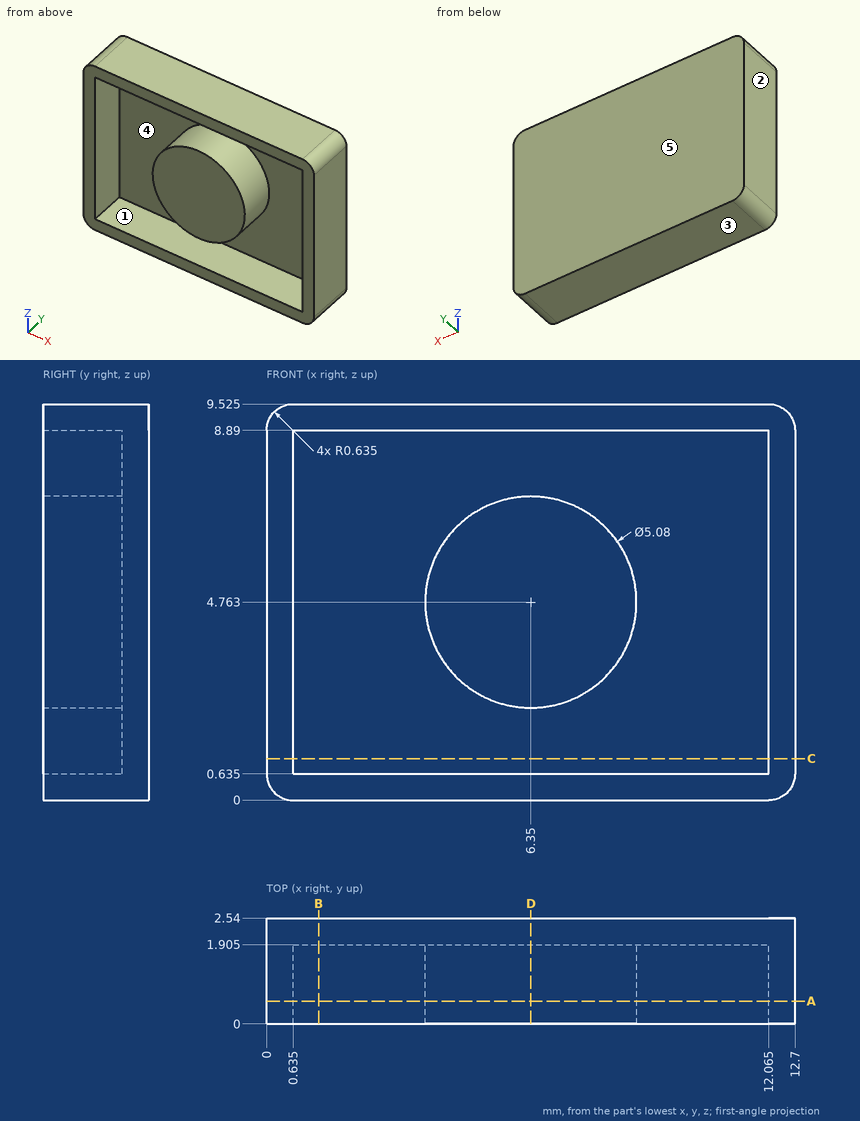
Print and shaded views of the part. All mm, measured from the part's lowest x, y and z. A direction names the side the tool comes from. Give positions to 0.01 mm unless a question says otherwise; leave off trailing zeros. Write each loop counter-clockwise with the first axis right and the second up, starting at its lowest first coordinate (ties: lowest second). Pieces come first, ordered by that corner, then holes. Notation, with made-up numbers: (-33.5, 82) -> (-12.5, 82) arc R16 cw to (-12.5, 108) -> close; hole circle Ø9 at (52, -40). An arc over 180 degrees is marked (long way). Write item = value, one per line.
(1) Slice it at C-C, the plane z = 1. Give the cut face in (x, y) (1 decimal).
Determined:
outline = (0, 0) -> (0.6, 0) -> (0.6, 1.9) -> (12.1, 1.9) -> (12.1, 0) -> (12.7, 0) -> (12.7, 2.5) -> (0, 2.5) -> close
(2) Slice it at A-A, the plane y = 0.55. Give the number of separate pieces and of enclosed holes in the cut face.
Determined:
separate_pieces = 2
enclosed_holes = 1
(3) Slice it at B-B, the plane x = 1.25. Give the cut face in (y, z) (1 decimal).
Determined:
outline = (0, 0) -> (2.5, 0) -> (2.5, 9.5) -> (0, 9.5) -> (0, 8.9) -> (1.9, 8.9) -> (1.9, 0.6) -> (0, 0.6) -> close
(4) Tool access for the marked faces 1 and 2: list every direction of +Z, -Z, +X, -X, +Y, -Y with a clear straight run to the whole face (end or side of a thin tool).
Determined:
face_1 = -Y
face_2 = +Z, -Z, -X, +Y, -Y
(5) Mould opens along Z. For the marked faces 3, 4 and 5 say: released by +Z, released by -Z, zero draft, split by the parting line, or undercut.
Determined:
face_3 = released by -Z
face_4 = undercut
face_5 = zero draft
(6) Probe line 1 along X through (y, z) = (0.75, 1) (1 decimal); line 2 along Z through (x, y) = (10, 1.35) (1 decimal); line 3 along Z through (x, y) = (8, 1.55) (1 decimal). List the from-to ranges inside material, lowest first.
Determined:
line_1 = 0 to 0.6, 12.1 to 12.7
line_2 = 0 to 0.6, 8.9 to 9.5
line_3 = 0 to 0.6, 2.8 to 6.7, 8.9 to 9.5
(7) Slice it at D-D, the plane x = 6.35. Give the cut face in (y, z) (1 decimal).
Determined:
outline = (0, 0) -> (2.5, 0) -> (2.5, 9.5) -> (0, 9.5) -> (0, 8.9) -> (1.9, 8.9) -> (1.9, 7.3) -> (0, 7.3) -> (0, 2.2) -> (1.9, 2.2) -> (1.9, 0.6) -> (0, 0.6) -> close
